from build123d import *

# Parameters (mm, degrees)
SKETCH_1_R               = 6
EXTRUDE_1_DEPTH          = 25
CUT_EXTRUDE_1_DEPTH      = 41.311288741
CUT_EXTRUDE_1_DEPTH_BACK = 41.311288741
SKETCH_2_W               = 21.902921801
SKETCH_2_H               = 31.191688498
SKETCH_2_W_2             = 23.513880173
SKETCH_2_H_2             = 33.775615356
CUT_EXTRUDE_2_REACH      = 45.875
CUT_EXTRUDE_2_END_RADIUS = 6
SKETCH_3_R               = 2.5
SKETCH_4_R               = 3
CUT_EXTRUDE_3_DEPTH      = 12
SKETCH_5_R               = 5.5
CUT_EXTRUDE_4_DEPTH      = 5
SKETCH_6_R               = 3
CUT_EXTRUDE_5_DEPTH      = 39.131352027
FILLET_1_R               = 1


with BuildPart() as part:
    # Эскиз1 → Бобышка-Вытянуть1 (new, symmetric)
    with BuildSketch(Plane.XY):
        with BuildLine():
            Line((-10, 0), (10, 0))
            Line((10, 0), (10, 20))
            ThreePointArc((10, 20), (0, 30), (-10, 20))
            Line((-10, 20), (-10, 0))
        make_face()
        with Locations((0, 20)):
            Circle(SKETCH_1_R, mode=Mode.SUBTRACT)
    extrude(amount=EXTRUDE_1_DEPTH, both=True)

    # Эскиз2 → Вырез-Вытянуть1 (cut, two sides: drawn at the far end of the back side and taken through both)
    with BuildSketch(Plane(origin=(0, 0, 0), x_dir=(0, 0, -1), z_dir=(1, 0, 0)).offset(-CUT_EXTRUDE_1_DEPTH_BACK)):
        with Locations((21.951460901, 23.595844249)):
            Rectangle(SKETCH_2_W, SKETCH_2_H)
        with Locations((-22.756940087, 24.887807678)):
            Rectangle(SKETCH_2_W_2, SKETCH_2_H_2)
    extrude(amount=CUT_EXTRUDE_1_DEPTH + CUT_EXTRUDE_1_DEPTH_BACK, mode=Mode.SUBTRACT)

    # Вырез-Вытянуть2: up to this cylinder (the profile starts outside it)
    cut_extrude_2_end = Plane(origin=(0, 20, 0), z_dir=(0, 0, -1)) * Cylinder(CUT_EXTRUDE_2_END_RADIUS, 104.75, mode=Mode.PRIVATE)
    # Эскиз3 → Вырез-Вытянуть2 (cut, up to the surface)
    with BuildSketch(Plane.ZY.offset(10), mode=Mode.PRIVATE) as cut_extrude_2_sk1:
        with Locations((0, 20)):
            Circle(SKETCH_3_R)
    cut_extrude_2_tool1 = extrude(cut_extrude_2_sk1.sketch, amount=-CUT_EXTRUDE_2_REACH, mode=Mode.PRIVATE) - cut_extrude_2_end
    add(cut_extrude_2_tool1.solids().sort_by_distance((-10, 20, 0))[0], mode=Mode.SUBTRACT)

    # Эскиз4 → Вырез-Вытянуть3 (cut)
    with BuildSketch(Plane(origin=(0, 0, 0), x_dir=(-1, 0, 0), z_dir=(0, -1, 0))):
        with Locations(Location((0, 0, 0), (0, 0, 90))):
            Circle(SKETCH_4_R)
    extrude(amount=-CUT_EXTRUDE_3_DEPTH, mode=Mode.SUBTRACT)

    # Эскиз5 → Вырез-Вытянуть4 (cut)
    with BuildSketch(Plane(origin=(0, 8, 0), x_dir=(1, 0, 0), z_dir=(0, 1, 0))):
        with Locations(Location((0, 17.5, 0), (0, 0, 270))):
            Circle(SKETCH_5_R)
        with Locations(Location((0, -17.5, 0), (0, 0, 270))):
            Circle(SKETCH_5_R)
    extrude(amount=-CUT_EXTRUDE_4_DEPTH, mode=Mode.SUBTRACT)

    # Эскиз6 → Вырез-Вытянуть5 (cut, through all)
    with BuildSketch(Plane(origin=(0, 3, 0), x_dir=(1, 0, 0), z_dir=(0, 1, 0))):
        with Locations(Location((0, 17.5, 0), (0, 0, 270))):
            Circle(SKETCH_6_R)
        with Locations(Location((0, -17.5, 0), (0, 0, 270))):
            Circle(SKETCH_6_R)
    extrude(amount=-CUT_EXTRUDE_5_DEPTH, mode=Mode.SUBTRACT)

    # Скругление1
    fillet_1_edges = [part.edges().sort_by_distance(p)[0] for p in [
        (10, 4, 25),
        (-10, 4, -25),
        (-10, 4, 25),
        (-10, 8, -18),
        (0, 8, -25),
        (10, 8, -18),
        (10, 14, -11),
        (0, 30, -11),
        (-10, 14, -11),
        (0, 8, 25),
        (-10, 14, 11),
        (0, 30, 11),
        (-10, 8, 18),
        (10, 8, 18),
        (10, 14, 11),
        (10, 4, -25),
    ]]
    fillet(fillet_1_edges, radius=FILLET_1_R)


solid = part.part
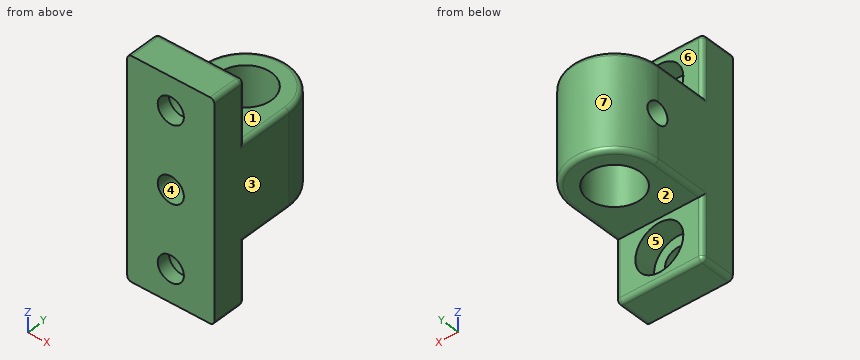
Here's how the part is built. I have some questions about the finished solid (model axes, mm). Face numbers are marked on the shaded views. A direction names the side the tool comes from. Coordinates: 2 decimals unless noted, no trailing zeros. Order: outer loops, then holes, each group sorted by start corner. A loop starts at its lowest first (then second) coordinate and runs counter-clockwise, first axis right, second up. Notation, with made-up numbers: M 4.25,51.25 L 49.25,51.25 A22 cw 49.25,89.25 Z; hole C 61,68.25 d6. An arc over 180 degrees is marked long. Answer as CSV lines item,"result".
Item 1: For pin 1 (5.5 mm diameter, centred on x = -0.5, z = -18.5, fed in from +Y); pin 2 (4 mm diameter, centred on y = 20, z = 0, fed in from -X); pin 3 (1.5 mm diameter, centred on x = 7, z = -17.5, fed in from +Y); pin 4 (8 mm diameter, centred on x = 2.5, z = 4.5, fed in from -Y), each with a flat end and sliding along its axis, tell me the tip position at first contact or that it passes through.
Results found:
pin 1,"y = 3"
pin 2,"x = 5.66"
pin 3,"y = 8"
pin 4,"y = 0"
Item 2: Imagine slicing it at A-A on z = 17.5. Write out the boundary of the cut face in (x, y), plus the area to 3 significant figures.
Results found:
outline,"M -10,0 L -3,0 L -3,3 L -5.5,3 L -5.5,8 L -9,8 A1 ccw -10,7 Z; M 3,0 L 10,0 L 10,7 A1 ccw 9,8 L 5.5,8 L 5.5,3 L 3,3 Z"
area,"86.6 mm2"
Item 3: We'd pull the mould along X, two halves only. Please class the marked faces 4, 5, 6 and 7: +X half, -X half, draft (parallel to the pull), parting line (faces both ways), or undercut.
Results found:
face 4,"undercut"
face 5,"undercut"
face 6,"draft"
face 7,"parting line"
Item 4: Imagine slicing it at B-B on y = 11. Write out the boundary of the cut face in (x, z).
Results found:
outline,"M -10,-10 A1 ccw -9,-11 L 9,-11 A1 ccw 10,-10 L 10,10 A1 ccw 9,11 L -9,11 A1 ccw -10,10 Z; hole C 0,0 d6"
Item 5: Imagine slicing it at C-C on z = 3.5. Write out the boundary of the cut face in (x, y).
Results found:
outline,"M -10,0 L 10,0 L 10,20 A10 ccw -10,20 Z; hole C 0,20 d12"
Item 6: Imagine slicing it at D-D on y = 19.5. Write out the boundary of the cut face in (x, z), plus the area to 3 significant figures.
Results found:
outline,"M -10,-10 A1 ccw -9,-11 L -5.98,-11 L -5.98,-2.45 L -10,-2.45 Z; M -10,2.45 L -5.98,2.45 L -5.98,11 L -9,11 A1 ccw -10,10 Z; M 5.98,-11 L 9,-11 A1 ccw 10,-10 L 10,10 A1 ccw 9,11 L 5.98,11 Z"
area,"156 mm2"
Item 7: On a 3-axis mill with a long thin cutter (end or side, diameter ignored), from which of +Z, -Z, +X, -X, +Y, -Y can I reach the whole of each face in a straight line? I mean the marked faces 1, 2 and 3. Say none if no direction works.
Results found:
face 1,"+Z, +X, -X, +Y"
face 2,"-Z, +X, -X, +Y"
face 3,"+Z, -Z, +X, +Y, -Y"
Item 8: If I drill on line 1 (Y direction, x = 0, z = -6.5); line 2 (Z direction, x = -8.6, y = 20); line 3 (X direction, y = 3, z = 0), over which ranges is the centre line in solid material (lowest first)?
Results found:
line 1,"0 to 14, 26 to 30"
line 2,"-11 to -2.5, 2.5 to 11"
line 3,"-10 to -3, 3 to 10"
